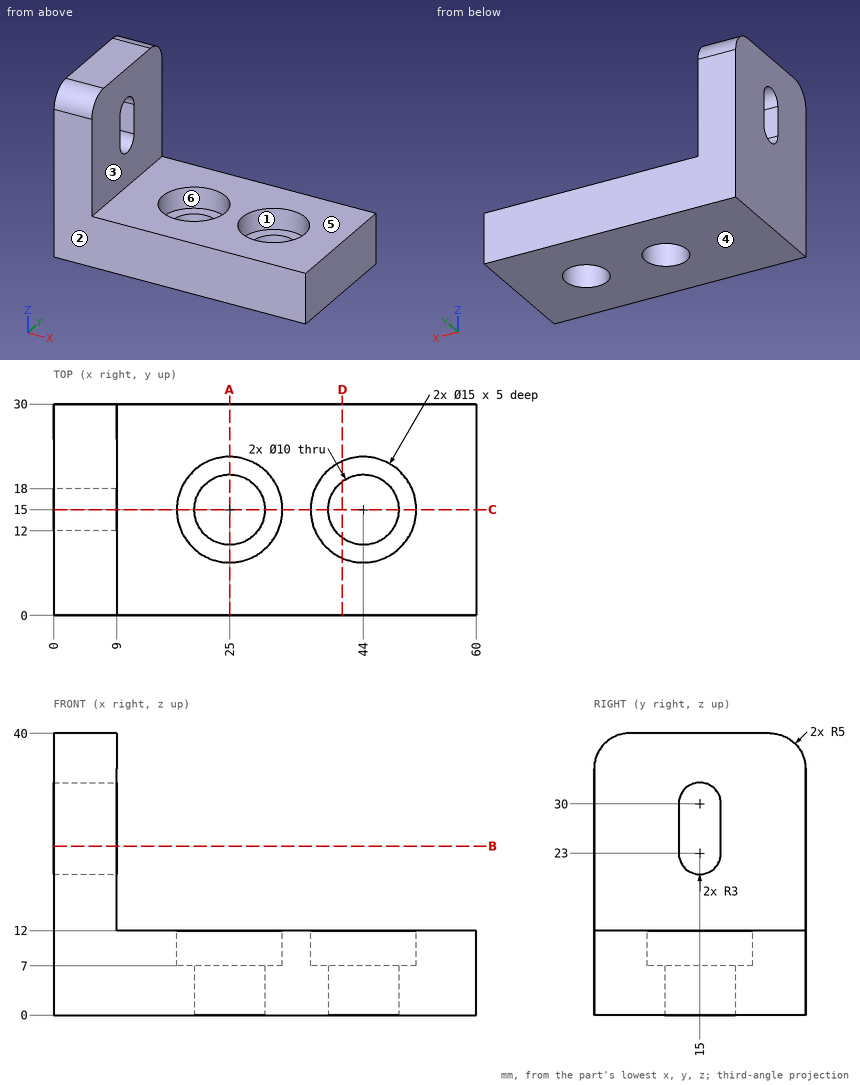
Can you work these out from the drawing? Everything is in mm from the part's minimum corner. A direction names the side the tool comes from. Give positions to 0.01 mm unless a question says otherwise; leave off trailing zeros. Loops run counter-clockwise (first coordinate to the right, second up) from the corner with the lowest first, then second, coordinate; pieces in that order, holes last. Notation, with made-up numbers: (-36.75, 25.25) -> (-18.75, 25.25) arc R13 ccw to (-18.75, 40.25) -> close; hole circle Ø9 at (34, 7.25). An arc over 180 degrees is marked (long way). Return JSON: item names as keys, results as strings.
Item 1: If we section it at D-D on x = 41: List the corners of the cut face in (y, z) for me.
Geometry results:
{"outline": "(0, 0) -> (11, 0) -> (11, 7) -> (8.13, 7) -> (8.13, 12) -> (0, 12) -> close; (19, 0) -> (30, 0) -> (30, 12) -> (21.87, 12) -> (21.87, 7) -> (19, 7) -> close"}
Item 2: If we section it at A-A on x = 25: List the corners of the cut face in (y, z) for me, plus the area to 3 significant figures.
Geometry results:
{"outline": "(0, 0) -> (10, 0) -> (10, 7) -> (7.5, 7) -> (7.5, 12) -> (0, 12) -> close; (20, 0) -> (30, 0) -> (30, 12) -> (22.5, 12) -> (22.5, 7) -> (20, 7) -> close", "area": "215 mm²"}
Item 3: I need wall thicknesses on L1, parallel to Y at x = 44, z = 3.5; L2, parallel to Y at x = 44, z = 10; L3, parallel to X at y = 3.5, z = 19. Which ranges of each line are inside material? Lowest first, please. Write a range as from..to.
Geometry results:
{"L1": "y = 0..10, 20..30", "L2": "y = 0..7.5, 22.5..30", "L3": "x = 0..9"}
Item 4: I'm going to push flat-ended pins straight in: pin 1 (12 mm diameter, centred on x = 43, y = 7, fed in from +Z); pin 2 (13.5 mm diameter, centred on x = 25, y = 15, fed in from +Z); pin 3 (14 mm diameter, centred on y = 11, z = 22.5, fed in from +X). Where does each tip first touch, or does it pass through?
Geometry results:
{"pin 1": "stops at z = 12", "pin 2": "stops at z = 7", "pin 3": "stops at x = 9"}
Item 5: We'd pull the mould along Y, two halves only. Please class the marked faces 1, 2 and 3: +Y half, -Y half, draft (parallel to the pull), parting line (faces both ways), or undercut.
Geometry results:
{"face 1": "undercut", "face 2": "-Y half", "face 3": "draft"}
Item 6: Which directions (+Z, -Z, +X, -X, +Y, -Y) give clear straight access to the entire face, cutting with the end or side of a thin tool? Please do the marked faces 4, 5 and 6.
Geometry results:
{"face 4": "-Z, +X, -X, +Y, -Y", "face 5": "+Z, +X, +Y, -Y", "face 6": "+Z"}
Item 7: If we section it at B-B on z = 24: List the corners of the cut face in (x, y) for me, plus the area to 3 significant figures.
Geometry results:
{"outline": "(0, 0) -> (9, 0) -> (9, 12) -> (0, 12) -> close; (0, 18) -> (9, 18) -> (9, 30) -> (0, 30) -> close", "area": "216 mm²"}
Item 8: If we section it at C-C on y = 15: List the corners of the cut face in (x, z) for me.
Geometry results:
{"outline": "(0, 0) -> (20, 0) -> (20, 7) -> (17.5, 7) -> (17.5, 12) -> (9, 12) -> (9, 20) -> (0, 20) -> close; (0, 33) -> (9, 33) -> (9, 40) -> (0, 40) -> close; (30, 0) -> (39, 0) -> (39, 7) -> (36.5, 7) -> (36.5, 12) -> (32.5, 12) -> (32.5, 7) -> (30, 7) -> close; (49, 0) -> (60, 0) -> (60, 12) -> (51.5, 12) -> (51.5, 7) -> (49, 7) -> close"}
